Read the model definition and answer for the solid it produces. Units are mm, in the model's axes. A direction names the side the tool comes from. Coordinates: 2 decimals unless noted, no trailing zeros. Loops run counter-clockwise (first coordinate to the right, second up) from the corner with the lowest first, then second, coordinate; pieces in that order, holes last.
from build123d import *

# Parameters (mm, degrees)
F1_DEPTH = 25
F2_DEPTH = 25


with BuildPart() as f1:
    # F0 (on Top) → F1 (new body)
    with BuildSketch(Plane.XY):
        with BuildLine():
            Line((20.510751, -26.791588), (20.510751, 43.208412))
            ThreePointArc((20.510751, 43.208412), (19.632072, 45.329732), (17.510751, 46.208412))
            Line((17.510751, 46.208412), (6.510751, 46.208412))
            Line((6.510751, 46.208412), (6.510751, 37.556949))
            ThreePointArc((6.510751, 37.556949), (6.126233, 36.554103), (5.169818, 36.065407))
            Line((5.169818, 36.065407), (-36.143343, 31.65953))
            Line((-36.143343, 31.65953), (-36.143343, 24.842082))
            Line((-36.143343, 24.842082), (-50.143343, 24.842082))
            Line((-50.143343, 24.842082), (-50.143343, 31.103174))
            Line((-50.143343, 31.103174), (-82.081185, 24.840478))
            ThreePointArc((-82.081185, 24.840478), (-83.814669, 23.809757), (-84.503856, 21.914401))
            Line((-84.503856, 21.914401), (-84.661583, -4.582726))
            ThreePointArc((-84.661583, -4.582726), (-83.961607, -6.526754), (-82.170625, -7.55709))
            Line((-82.170625, -7.55709), (-49.996673, -13.096121))
            Line((-49.996673, -13.096121), (-49.996673, -7.157918))
            Line((-49.996673, -7.157918), (-35.996673, -7.157918))
            Line((-35.996673, -7.157918), (-35.996673, -13.816103))
            Line((-35.996673, -13.816103), (5.219561, -19.610079))
            ThreePointArc((5.219561, -19.610079), (6.142832, -20.111405), (6.510751, -21.095474))
            Line((6.510751, -21.095474), (6.510751, -29.791588))
            Line((6.510751, -29.791588), (17.510751, -29.791588))
            ThreePointArc((17.510751, -29.791588), (19.632072, -28.912909), (20.510751, -26.791588))
        make_face()
    extrude(amount=F1_DEPTH)

    # F0 (on Top) → F2 (join)
    with BuildSketch(Plane.XY):
        with BuildLine():
            Line((20.510751, -26.791588), (20.510751, 43.208412))
            ThreePointArc((20.510751, 43.208412), (19.632072, 45.329732), (17.510751, 46.208412))
            Line((17.510751, 46.208412), (6.510751, 46.208412))
            Line((6.510751, 46.208412), (6.510751, 37.556949))
            ThreePointArc((6.510751, 37.556949), (6.126233, 36.554103), (5.169818, 36.065407))
            Line((5.169818, 36.065407), (-36.143343, 31.65953))
            Line((-36.143343, 31.65953), (-36.143343, 24.842082))
            Line((-36.143343, 24.842082), (-50.143343, 24.842082))
            Line((-50.143343, 24.842082), (-50.143343, 31.103174))
            Line((-50.143343, 31.103174), (-82.081185, 24.840478))
            ThreePointArc((-82.081185, 24.840478), (-83.814669, 23.809757), (-84.503856, 21.914401))
            Line((-84.503856, 21.914401), (-84.661583, -4.582726))
            ThreePointArc((-84.661583, -4.582726), (-83.961607, -6.526754), (-82.170625, -7.55709))
            Line((-82.170625, -7.55709), (-49.996673, -13.096121))
            Line((-49.996673, -13.096121), (-49.996673, -7.157918))
            Line((-49.996673, -7.157918), (-35.996673, -7.157918))
            Line((-35.996673, -7.157918), (-35.996673, -13.816103))
            Line((-35.996673, -13.816103), (5.219561, -19.610079))
            ThreePointArc((5.219561, -19.610079), (6.142832, -20.111405), (6.510751, -21.095474))
            Line((6.510751, -21.095474), (6.510751, -29.791588))
            Line((6.510751, -29.791588), (17.510751, -29.791588))
            ThreePointArc((17.510751, -29.791588), (19.632072, -28.912909), (20.510751, -26.791588))
        make_face()
    extrude(amount=F2_DEPTH)


solid = f1.part
Item 1: A cutting plane is placed at D-D on x = -55. Determine the outline of the cut face in (y, z).
Numbers:
outline: (-12.23, 0) - (30.15, 0) - (30.15, 25) - (-12.23, 25) - close
Item 2: Which of the six approach directions +Z, -Z, +X, -X, +Y, -Y give full straight-line access (tool end or side, diameter ignored) to faces 1 (the face through (6.511, 42, 12)), 2 (the face through (-49.997, -10, 12)), 3 (the face through (6.511, -25, 12))?
Numbers:
face 1: +Z, -Z, -X, +Y
face 2: +Z, -Z, -Y
face 3: +Z, -Z, -X, -Y
Item 3: Determine the mould class of faces 4 (the face through (-15.198, 33.893, 12.325)), 5 (the face through (19.609, -28.936, 12.325)), 6 (the face through (-43, 24.842, 12)), 7 (the face through (-36.143, 28, 12)) for opening direction X: released by +X, released by -X, zero draft, split by the parting line, or undercut.
Numbers:
face 4: released by -X
face 5: released by +X
face 6: undercut
face 7: undercut
Item 4: A cutting plane is placed at B-B on z = 19.25. Determine the outline of the cut face in (x, y).
Numbers:
outline: (-84.66, -4.58) arc R3 ccw to (-82.17, -7.56) - (-50, -13.1) - (-50, -7.16) - (-36, -7.16) - (-36, -13.82) - (5.22, -19.61) arc R1.5 cw to (6.51, -21.1) - (6.51, -29.79) - (17.51, -29.79) arc R3 ccw to (20.51, -26.79) - (20.51, 43.21) arc R3 ccw to (17.51, 46.21) - (6.51, 46.21) - (6.51, 37.56) arc R1.5 cw to (5.17, 36.07) - (-36.14, 31.66) - (-36.14, 24.84) - (-50.14, 24.84) - (-50.14, 31.1) - (-82.08, 24.84) arc R3 ccw to (-84.5, 21.91) - close
Item 5: Find the intervals of material crossed by line 1 along X through (y, z) = (0, 5.5); line 2 along Y through (x, z) = (-39.5, 14.5); line 3 along X through (y, z) = (-3, 7.25), in increasing order.
Numbers:
line 1: x = -84.63 to 20.51
line 2: y = -7.16 to 24.84
line 3: x = -84.65 to 20.51
Item 6: A cutting plane is placed at A-A on y = -12. Determine the outline of the cut face in (x, z), then the cut area to 3 significant figures.
Numbers:
outline: (-56.36, 0) - (-50, 0) - (-50, 25) - (-56.36, 25) - close; (-36, 0) - (20.51, 0) - (20.51, 25) - (-36, 25) - close
area: 1,570 mm2
Item 7: Given pin 1 (9.5 mm diameter, centred on y = -27, z = 14.5, fed in from -X); pin 2 (11 mm diameter, centred on x = -43, z = 6.5, fed in from +Y); pin 3 (7.5 mm diameter, centred on y = -10, z = 10, fed in from -X), each flat-ended and moving along its own axis, determine where each tip first touches the part or whether it passes through.
Numbers:
pin 1: stops at x = 6.51
pin 2: stops at y = 24.84
pin 3: stops at x = -84.17
Item 8: A cutting plane is placed at C-C on x = -43. Determine the outline of the cut face in (y, z).
Numbers:
outline: (-7.16, 0) - (24.84, 0) - (24.84, 25) - (-7.16, 25) - close
